Verification items for the finished model (mm, model axes). A direction names the side the tool comes from. Give positions to 0.01 mm unless a question says otherwise; leave off trailing zeros. Order: outer loops, then holes, each group sorted by start corner. A loop starts at its lowest first (then second) coordinate and runs counter-clockwise, first axis right, second up.
(1) Sectioned sample at A-A on z = 1.45. Record the cut outline in (x, y), plus the area to 3 significant figures.
(2) Access from +Z, -Z, +X, -X, +Y, -Y to the whole of each face (thin tool, end or side, straight path). Record for faces 1 (the face through (43, 3, 2)), 2 (the face through (67, 9.5, 2)).
(3) Scan lines: L1, parallel to Y at x = 18.5, z = 2.4; L2, parallel to X at y = 2.5, z = 3.45; L3, parallel to X at y = 1.5, z = 2.6. Record each from-to range of solid material in increasing order.
(4) Gauge pin test, flat ends, axial feed: pin 1 (1.1 mm diameter, centred on y = 0.5, z = 3.5, fed in from +X); pin 2 (1.5 mm diameter, centred on x = 36.5, y = 1.5, fed in from +Z). Record the tip position at first contact, or that the pin passes through.
(5) Sectioned sample at B-B on x = 54. Record the cut outline in (y, z).
```python
from build123d import *

# Parameters (mm, degrees)
BOSS_EXTRUDE1_DEPTH = 5
SKETCH3_W           = 0.1
SKETCH3_H           = 5
CUT_EXTRUDE1_DEPTH  = 3


with BuildPart() as part:
    # Sketch1 → Boss-Extrude1 (new body)
    with BuildSketch(Plane.XY):
        with BuildLine():
            Line((0, 0), (0, 7.5))
            ThreePointArc((0, 7.5), (0.585786438, 8.914213562), (2, 9.5))
            Line((2, 9.5), (69, 9.5))
            ThreePointArc((69, 9.5), (69.707106781, 9.207106781), (70, 8.5))
            Line((70, 8.5), (70, 4))
            ThreePointArc((70, 4), (69.707106781, 3.292893219), (69, 3))
            Line((69, 3), (17, 3))
            ThreePointArc((17, 3), (15.585786438, 2.414213562), (15, 1))
            Line((15, 1), (15, 0))
            Line((15, 0), (11, 0))
            Line((11, 0), (4, 0))
            Line((4, 0), (0, 0))
        make_face()
    extrude(amount=BOSS_EXTRUDE1_DEPTH)

    # Sketch3 → Cut-Extrude1 (cut)
    with BuildSketch(Plane(origin=(0, 9.5, 0), x_dir=(1, 0, 0), z_dir=(0, 1, 0))):
        with Locations((64.95, -2.5)):
            Rectangle(SKETCH3_W, SKETCH3_H)
    extrude(amount=-CUT_EXTRUDE1_DEPTH, mode=Mode.SUBTRACT)


solid = part.part
```
Ans:
1. outline: (0, 0) - (15, 0) - (15, 1) arc R2 cw to (17, 3) - (69, 3) arc R1 ccw to (70, 4) - (70, 8.5) arc R1 ccw to (69, 9.5) - (65, 9.5) - (65, 6.5) - (64.9, 6.5) - (64.9, 9.5) - (2, 9.5) arc R2 ccw to (0, 7.5) - close
1. area: 499 mm2
2. face 1: +Z, -Z, +X, -Y
2. face 2: +Z, -Z, +X, -X, +Y
3. L1: y = 3 to 9.5
3. L2: x = 0 to 15.68
3. L3: x = 0 to 15.06
4. pin 1: stops at x = 15
4. pin 2: passes through
5. outline: (3, 0) - (9.5, 0) - (9.5, 5) - (3, 5) - close
